from build123d import *

# Parameters (mm, degrees)
SKETCH_1_R          = 2
EXTRUDE_1_DEPTH     = 5
SKETCH_2_R          = 3
EXTRUDE_2_DEPTH     = 10
EXTRUDE_START       = 4.5
EXTRUDE_3_DEPTH     = 4.5
CUT_EXTRUDE_1_DEPTH = 4.5


with BuildPart() as part:
    # 草图1 → 凸台-拉伸1 (new body)
    with BuildSketch(Plane(origin=(0, 0, 0), x_dir=(1, 0, 0), z_dir=(0, 1, 0))):
        with BuildLine():
            Line((0, 10), (100, 10))
            ThreePointArc((100, 10), (110, 0), (100, -10))
            Line((100, -10), (0, -10))
            ThreePointArc((0, -10), (-10, 0), (0, 10))
        make_face()
        with Locations(Location((0, 0, 0), (0, 0, 270))):
            Circle(SKETCH_1_R, mode=Mode.SUBTRACT)
    extrude(amount=EXTRUDE_1_DEPTH)

    # 草图2 → 凸台-拉伸2 (add)
    with BuildSketch(Plane(origin=(0, 5, 0), x_dir=(1, 0, 0), z_dir=(0, 1, 0))):
        with Locations(Location((100, 0, 0), (0, 0, 270))):
            Circle(SKETCH_2_R)
    extrude(amount=EXTRUDE_2_DEPTH)

    # 草图3 → 凸台-拉伸3 (add)
    with BuildSketch(Plane.XZ.offset(EXTRUDE_START)):
        with BuildLine():
            Line((100, 10), (73.40776322, 10))
            Line((73.40776322, 10), (73.40776322, -10))
            Line((73.40776322, -10), (100, -10))
            ThreePointArc((100, -10), (110, 0), (100, 10))
        make_face()
    extrude(amount=-EXTRUDE_3_DEPTH)

    # 草图4 → 切除-拉伸1 (cut)
    with BuildSketch(Plane.XZ.offset(4.5)):
        with BuildLine():
            Line((79.849230428, 2.288593229), (99.690178504, 3.236180981))
            ThreePointArc((99.690178504, 3.236180981), (103.250977807, 0), (99.690178504, -3.236180981))
            Line((99.690178504, -3.236180981), (79.849230428, -2.288593229))
            ThreePointArc((79.849230428, -2.288593229), (77.560637199, 0), (79.849230428, 2.288593229))
        make_face()
    extrude(amount=-CUT_EXTRUDE_1_DEPTH, mode=Mode.SUBTRACT)


solid = part.part
The listing builds one solid part. Answer for the finished solid, in the listing's coordinates (mm). A direction names the side the tool comes from. Coordinates: 2 decimals unless noted, no trailing zeros. Loops run counter-clockwise (first coordinate to the right, second up) from the corner with the lowest first, then second, coordinate; pieces in that order, holes last. Notation, with made-up numbers: (86.5, 77) -> (102.5, 77) arc R26 ccw to (102.5, 104) -> close; hole circle Ø7 at (-33, 8). An arc over 180 degrees is marked (long way). Answer in a Markdown table with one row per item. Add a question column.
1. The part is cut by section A-A, the plane z = 0. Write down the section's boundary in (x, y).
2. Flat-ended cylindrical pins translate along their axes: P1, Ø8, axis at x = 19, z = 7, coming from the -Y side; P2, Ø8, axis at x = 88, z = 4.5, coming from the +Y side; P3, Ø8, axis at y = 1, z = 5, coming from the +X side. Find the tip coordinate at first contact, or state that the pin passes through.
3. For faces 1 (the cylindrical face through (97.07, 9.93, -0.65)), 2 (the cylindrical face through (77.56, -2.28, -0.05)), 3 (the flat face through (100, 15, 0)), 4 (the flat face through (73.408, -2, 0)), 5 (the flat face through (91, -4.5, 5)), determine the directions among +Z, -Z, +X, -X, +Y, -Y from which every point of the face is accessible in a straight line to the end or side of a thin tool.
4. The part is cut by section C-C, the plane x = 98.5. Write down the section's boundary in (y, z), then the cut area to 3 significant figures.
5. The part is cut by section D-D, the plane z = 8.75. Write down the section's boundary in (x, y).
6. The part is cut by section B-B, the plane y = 1.25. Write down the section's boundary in (x, z), then the cut area to 3 significant figures.
7. Consider line 1 (X direction, y = 2.25, z = 0); line 2 (Z direction, x = 100, y = -1.8); line 3 (Y direction, x = 40, z = 7.75). Determine where each line is inside the solid, lowest interval first. Write a range as [from, to].
8. Determine the mould class of faces 6 (the flat face through (89.631, -2.282, 2.756)), 7 (the flat face through (60, 1, -10)), 8 (the cylindrical face through (-10, 2, 0)) for opening direction X: +X half, -X half, draft (parallel to the pull), parting line (faces both ways), or undercut.
Answer below:
| question | item | result |
|---|---|---|
| 1 | outline | (-10, 0) -> (-2, 0) -> (-2, 5) -> (-10, 5) -> close; (2, 0) -> (73.41, 0) -> (73.41, -4.5) -> (77.56, -4.5) -> (77.56, 0) -> (103.25, 0) -> (103.25, -4.5) -> (110, -4.5) -> (110, 5) -> (103, 5) -> (103, 15) -> (97, 15) -> (97, 5) -> (2, 5) -> close |
| 2 | P1 | y = 0 |
| 2 | P2 | y = 5 |
| 2 | P3 | x = 109.95 |
| 3 | face 1 | +Y |
| 3 | face 2 | -Y |
| 3 | face 3 | +Z, -Z, +X, -X, +Y |
| 3 | face 4 | +Z, -Z, -X, -Y |
| 3 | face 5 | +Z, -Z, +X, -X, -Y |
| 4 | outline | (-4.5, -10) -> (5, -10) -> (5, -2.6) -> (15, -2.6) -> (15, 2.6) -> (5, 2.6) -> (5, 10) -> (-4.5, 10) -> (-4.5, 3.18) -> (0, 3.18) -> (0, -3.18) -> (-4.5, -3.18) -> close |
| 4 | area | 213 mm2 |
| 5 | outline | (-4.84, 0) -> (73.41, 0) -> (73.41, -4.5) -> (104.84, -4.5) -> (104.84, 5) -> (-4.84, 5) -> close |
| 6 | outline | (0, -10) -> (100, -10) arc R10 ccw to (100, 10) -> (0, 10) arc R10 ccw to start; hole circle Ø4 at (0, 0) |
| 6 | area | 2,300 mm2 |
| 7 | line 1 | [-10, -2], [2, 110] |
| 7 | line 2 | [-10, -3.25], [3.25, 10] |
| 7 | line 3 | [0, 5] |
| 8 | face 6 | undercut |
| 8 | face 7 | draft |
| 8 | face 8 | -X half |
